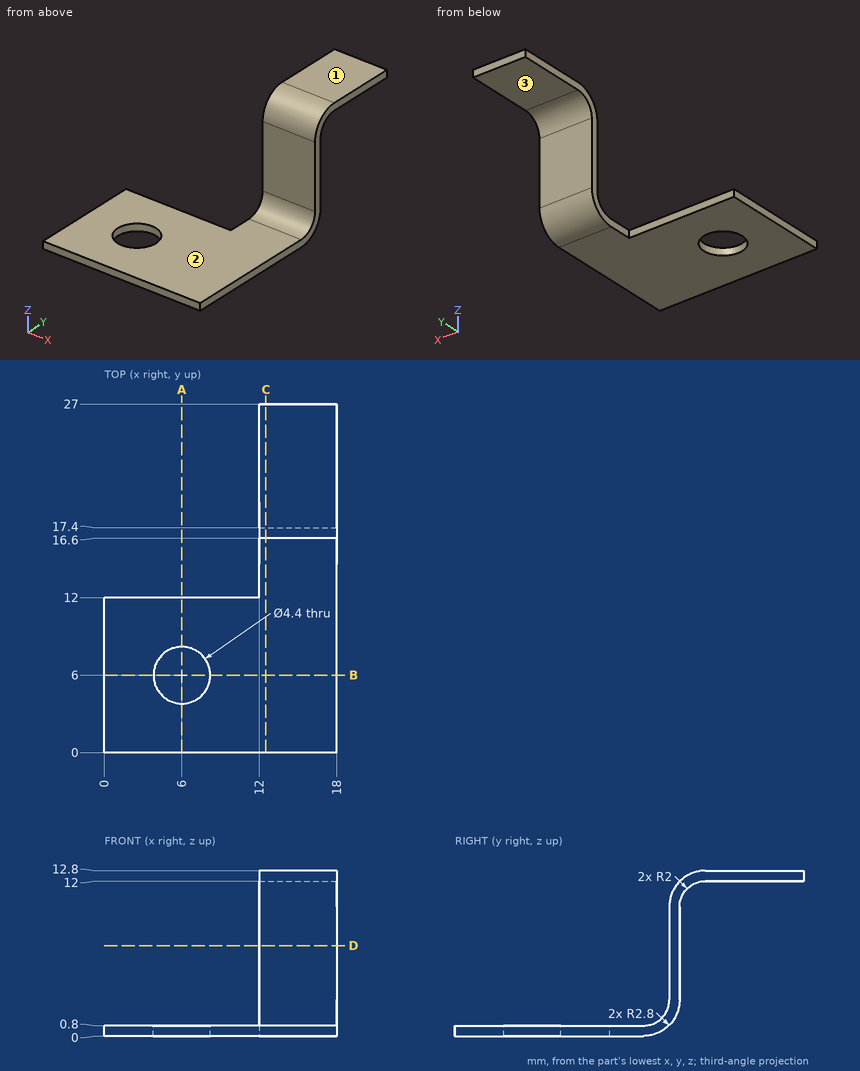
Here's the drawing with two shaded views (mm, measured from the low corner). I have some questions. A direction names the side the tool comes from. Give positions to 0.01 mm unless a question says otherwise; leave off trailing zeros. Write each loop counter-clockwise with the first axis right and the second up, starting at its lowest first coordinate (ties: lowest second). Pieces come first, ordered by that corner, then holes. Notation, with made-up numbers: (16, 77.5) -> (36, 77.5) arc R25 ccw to (36, 91.5) -> close; hole circle Ø8 at (14.25, 65.5). An arc over 180 degrees is marked (long way). Answer as a JSON object with one key per item and string values. Group by question number.
Item 1: Suppose I cut it at A-A (x = 6). Please give me the cut outline in (y, z), plus the area to 3 significant figures.
Item 2: Suppose I cut it at B-B (y = 6). Please give me the cut outline in (x, z), plus the area to 3 significant figures.
Item 3: Suppose I cut it at D-D (z = 7). Please give me the cut outline in (x, y), plus the area to 3 significant figures.
Item 4: I'm going to push flat-ended pins straight in: P1, Ø6.5, axis at x = 16, y = 25, coming from the -Z side; P2, Ø5, axis at x = 14, z = 5, coming from the -Y side; P3, Ø3, axis at x = 16, z = 6.5, coming from the +Y side. Where does each tip first touch, or does it pass through?
Item 5: Please list where these lines run through material, in increasing order: line 1 (X direction, y = 6, z = 0.2); line 2 (Y direction, x = 6, z = 0.5); line 3 (Z direction, x = 14, y = 11). Write a range as [from, to].
Item 6: Suppose I cut it at C-C (x = 12.5). Please give me the cut outline in (y, z).
Item 7: For the marked faces 1, 2 and 3, which set-ups out of +Z, -Z, +X, -X, +Y, -Y let a thin tool reach every point of the face, with its end or its side?
Findings:
{
 "1": {"outline": "(0, 0) -> (3.8, 0) -> (3.8, 0.8) -> (0, 0.8) -> close; (8.2, 0) -> (12, 0) -> (12, 0.8) -> (8.2, 0.8) -> close", "area": "6.08 mm²"},
 "2": {"outline": "(0, 0) -> (3.8, 0) -> (3.8, 0.8) -> (0, 0.8) -> close; (8.2, 0) -> (18, 0) -> (18, 0.8) -> (8.2, 0.8) -> close", "area": "10.9 mm²"},
 "3": {"outline": "(12, 16.6) -> (18, 16.6) -> (18, 17.4) -> (12, 17.4) -> close", "area": "4.80 mm²"},
 "4": {"P1": "stops at z = 12", "P2": "stops at y = 16.58", "P3": "stops at y = 17.4"},
 "5": {"line 1": "x = [0, 3.8], [8.2, 18]", "line 2": "y = [0, 3.8], [8.2, 12]", "line 3": "z = [0, 0.8]"},
 "6": {"outline": "(0, 0) -> (14.6, 0) arc R2.8 ccw to (17.4, 2.8) -> (17.4, 10) arc R2 cw to (19.4, 12) -> (27, 12) -> (27, 12.8) -> (19.4, 12.8) arc R2.8 ccw to (16.6, 10) -> (16.6, 2.8) arc R2 cw to (14.6, 0.8) -> (0, 0.8) -> close"},
 "7": {"face 1": "+Z, +X, -X, +Y, -Y", "face 2": "+Z, +X, -X, -Y", "face 3": "-Z, +X, -X, +Y"}
}
